from build123d import *

# Parameters (mm, degrees)
F0_W          = 85
F0_H          = 345
F1_DEPTH      = 42
F2_T          = -2
F3_W          = 81
F3_H          = 40
F4_DEPTH      = 172.5
F4_DEPTH_BACK = 172.5
F6_START      = 40
F5_W          = 15
F5_H          = 345
F6_DEPTH      = 2
F8_START      = -170.5
F7_W          = 81
F7_H          = 40
F8_DEPTH      = 2


with BuildPart() as f1:
    # F0 (on Top) → F1 (new body)
    with BuildSketch(Plane.XY):
        Rectangle(F0_W, F0_H)
    extrude(amount=F1_DEPTH)

    # F2
    f2_openings = [f1.faces().sort_by_distance(p)[0] for p in [
        (0, 0, 42),
    ]]
    offset(amount=F2_T, openings=f2_openings)

    # F3 (on Front) → F4 (cut, two sides)
    with BuildSketch(Plane.XZ) as f4_sk:
        with Locations((0, 22)):
            Rectangle(F3_W, F3_H)
    extrude(amount=F4_DEPTH, mode=Mode.SUBTRACT)
    extrude(f4_sk.sketch, amount=-F4_DEPTH_BACK, mode=Mode.SUBTRACT)

    # F5 (on Top) → F6 (join)
    with BuildSketch(Plane.XY.offset(F6_START)):
        with Locations((-50, 0)):
            Rectangle(F5_W, F5_H)
        with Locations((50, 0)):
            Rectangle(F5_W, F5_H)
    extrude(amount=F6_DEPTH)

    # F7 (on Front) → F8 (join)
    with BuildSketch(Plane.XZ.offset(F8_START)):
        with Locations((0, 22)):
            Rectangle(F7_W, F7_H)
    extrude(amount=-F8_DEPTH)


solid = f1.part
For this review, take the finished solid that the model builds, in its own axes (mm). A direction names the side the tool comes from. Round coordinates to 2 decimals unless told otherwise and drop trailing zeros. Write each loop counter-clockwise with the first axis right and the second up, starting at its lowest first coordinate (ties: lowest second). Pieces come first, ordered by that corner, then holes. Notation, with made-up numbers: (37.5, 42) - (73.5, 42) arc R29 cw to (73.5, 80) - close; hole circle Ø5 at (3, -23). An arc over 180 degrees is marked (long way). Write item = value, one per line. Start each with the question number.
1. Draft analysis for pull direction X (two halves, no side actions). For faces 6 (the face through (42.5, -2, 20)), 7 (the face through (21, -172.5, 1)), 8 (the face through (40.5, 1, 22)), 9 (the face through (-1, 1, 2)), state which applies: released by +X, released by -X, zero draft, split by the parting line, or undercut.
2. Consider section A-A on y = -12.5. State the section outline as (x, z) points, plus the area to 3 significant figures.
3. Wall thickness on L1, parallel to X at y = 29.5, z = 35; L2, parallel to Z at x = 26, y = 6.5; L3, parallel to Y at x = 11, z = 20.5: over which ranges is each line inside the solid? List them lowest first.
4. For faces 1 (the face through (-1, 170.5, 22)), 2 (the face through (-50, 2, 40)), 3 (the face through (50, 2, 40)), 4 (the face through (-43, -1, 42)), 5 (the face through (-1, 172.5, 21)), list the 3-axis set-ups (+Z, -Z, +X, -X, +Y, -Y) from which the entire face can be reached by the end or side of a thin tool; tool diameter is ignored.
5. Consider section C-C on z = 14. State the section outline as (x, y) points.
6. Consider section B-B on x = 6.5. State the section outline as (y, z) points.
7. Consider section D-D on x = 46. State the section outline as (y, z) points.
8. For pin 1 Ø2 at (y, z) = (128, 19.5) entering from -X; pin 2 Ø8 at (x, y) = (26.5, -41) entering from +Z; pin 3 Ø12 at (x, y) = (50.5, 27) entering from -Z; pin 4 Ø12 at (x, y) = (-9.5, -115) entering from -Z, all flat-tipped, find the tip position at first contact; note any pin that passes through.
Evaluation:
q1.face_6 = released by +X
q1.face_7 = zero draft
q1.face_8 = undercut
q1.face_9 = undercut
q2.outline = (-57.5, 40) - (-42.5, 40) - (-42.5, 0) - (42.5, 0) - (42.5, 40) - (57.5, 40) - (57.5, 42) - (40.5, 42) - (40.5, 2) - (-40.5, 2) - (-40.5, 42) - (-57.5, 42) - close
q2.area = 390 mm2
q3.L1 = -42.5 to -40.5, 40.5 to 42.5
q3.L2 = 0 to 2
q3.L3 = 170.5 to 172.5
q4.face_1 = +Z, -Y
q4.face_2 = -Z, -X, +Y, -Y
q4.face_3 = -Z, +X, +Y, -Y
q4.face_4 = +Z, +X, -X, +Y, -Y
q4.face_5 = +Z, -Z, +X, -X, +Y
q5.outline = (-42.5, -172.5) - (-40.5, -172.5) - (-40.5, 170.5) - (40.5, 170.5) - (40.5, -172.5) - (42.5, -172.5) - (42.5, 172.5) - (-42.5, 172.5) - close
q6.outline = (-172.5, 0) - (172.5, 0) - (172.5, 42) - (170.5, 42) - (170.5, 2) - (-172.5, 2) - close
q7.outline = (-172.5, 40) - (172.5, 40) - (172.5, 42) - (-172.5, 42) - close
q8.pin_1 = -42.5
q8.pin_2 = 2
q8.pin_3 = 40
q8.pin_4 = 0
